Geometry: final body of the model. Coordinates: model frame, mm. A direction names the side the tool comes from. Coordinates: 2 decimals unless noted, no trailing zeros. Write each loop counter-clockwise with the first axis right and the second up, starting at its lowest first coordinate (ties: lowest second). Pieces come first, ordered by that corner, then holes. Notation, with made-up numbers: (-2, 62) -> (53, 62) arc R7 cw to (53, 73) -> close; hole circle Ø5 at (-9, 75.25). An arc over 180 degrees is marked (long way). One line per item, written item: value.
```python
from build123d import *
from build123d.topology import SkipClean

# Parameters (mm, degrees)
BOSS_EXTRUDE1_DEPTH     = 15
SKETCH2_R               = 30
BOSS_EXTRUDE2_DEPTH     = 25
SKETCH3_R               = 20
SKETCH3_R_2             = 10
BOSS_EXTRUDE3_DEPTH     = 15
CUT_EXTRUDE1_DEPTH      = 146.344418537
CUT_EXTRUDE1_DEPTH_BACK = 146.344418537
SKETCH4_R               = 20
SKETCH5_R               = 10
BOSS_EXTRUDE4_DEPTH     = 25


with BuildPart() as part:
    # Sketch1 → Boss-Extrude1 (new body)
    with BuildSketch(Plane.YZ):
        with BuildLine():
            Line((-14.764588704, 87.647058824), (-29.529177407, 5.294117647))
            ThreePointArc((-29.529177407, 5.294117647), (0, -30), (29.529177407, 5.294117647))
            Line((29.529177407, 5.294117647), (14.764588704, 87.647058824))
            ThreePointArc((14.764588704, 87.647058824), (0, 100), (-14.764588704, 87.647058824))
        make_face()
    extrude(amount=BOSS_EXTRUDE1_DEPTH)

    # Sketch2 → Boss-Extrude2 (add)
    with BuildSketch(Plane.YZ.offset(15)):
        with Locations(Location((0, 0, 0), (0, 0, 10.164248622))):
            Circle(SKETCH2_R)
    extrude(amount=BOSS_EXTRUDE2_DEPTH)

    # Sketch3 → Boss-Extrude3 (add)
    with SkipClean():  # the faces are left unmerged after this step: merging them gives an invalid solid
        with BuildSketch(Plane.YZ.offset(40)):
            with BuildLine():
                Line((6, 29.393876913), (78, 14.696938457))
                ThreePointArc((78, 14.696938457), (90, 0), (78, -14.696938457))
                Line((78, -14.696938457), (6, -29.393876913))
                ThreePointArc((6, -29.393876913), (-30, 0), (6, 29.393876913))
            make_face()
            with Locations(Location((0, 0, 0), (0, 0, 270))):
                Circle(SKETCH3_R, mode=Mode.SUBTRACT)
            with Locations(Location((75, 0, 0), (0, 0, 270))):
                Circle(SKETCH3_R_2, mode=Mode.SUBTRACT)
        extrude(amount=BOSS_EXTRUDE3_DEPTH)

    # Sketch4 → Cut-Extrude1 (cut, two sides: drawn at the far end of the back side and taken through both)
    with SkipClean():  # the faces are left unmerged after this step: merging them gives an invalid solid
        with BuildSketch(Plane.YZ.offset(55).offset(-CUT_EXTRUDE1_DEPTH_BACK)):
            with Locations(Location((0, 0, 0), (0, 0, 270))):
                Circle(SKETCH4_R)
        extrude(amount=CUT_EXTRUDE1_DEPTH + CUT_EXTRUDE1_DEPTH_BACK, mode=Mode.SUBTRACT)

    # Sketch5 → Boss-Extrude4 (add)
    with SkipClean():  # the faces are left unmerged after this step: merging them gives an invalid solid
        with BuildSketch(Plane(origin=(0, 0, 0), x_dir=(0, -1, 0), z_dir=(-1, 0, 0))):
            with Locations(Location((0, 85, 0), (0, 0, 270))):
                Circle(SKETCH5_R)
        extrude(amount=BOSS_EXTRUDE4_DEPTH)


solid = part.part
```
(1) Section A-A (y = 0). Return the cut outline in (x, z).
Responses:
outline: (-25, 75) -> (0, 75) -> (0, 20) -> (55, 20) -> (55, 30) -> (15, 30) -> (15, 100) -> (0, 100) -> (0, 95) -> (-25, 95) -> close; (0, -30) -> (55, -30) -> (55, -20) -> (0, -20) -> close
(2) Section B-B (z = 0). Return the cut outline in (x, y), then the cut area to 3 significant figures.
Responses:
outline: (0, -30) -> (55, -30) -> (55, -20) -> (0, -20) -> close; (0, 20) -> (55, 20) -> (55, 65) -> (40, 65) -> (40, 30) -> (0, 30) -> close; (40, 85) -> (55, 85) -> (55, 90) -> (40, 90) -> close
area: 1,700 mm2
(3) Line query: line 1 (Y direction, x = 43, z = 0); line 2 (Z direction, x = 22, y = 0); line 3 (X direction, y = 67.5, z = -7). Output: solid intervals per line, ascending. Write a range as [from, to].
Responses:
line 1: y = [-30, -20], [20, 65], [85, 90]
line 2: z = [-30, -20], [20, 30]
line 3: x = [40, 55]
(4) Section D-D (x = 42). Return the cut outline in (y, z), then the cut area to 3 significant figures.
Responses:
outline: (6, -29.39) -> (78, -14.7) arc R15 ccw to (78, 14.7) -> (6, 29.39) arc R30 ccw (long way) to start; hole circle Ø40 at (0, 0); hole circle Ø20 at (75, 0)
area: 3,640 mm2
(5) Pull-direction query (Y, two-part tool) for faces 4 (the cylindrical face through (47.395, 84.915, 1.302)), 5 (the cylindrical face through (-12, 0, 95)), 6 (the flat face through (15, 0, 53)); classes: released by +Y, released by -Y, zero draft, split by the parting line, or undercut.
Responses:
face 4: undercut
face 5: split by the parting line
face 6: zero draft
(6) Section C-C (x = 2.5). Return the cut outline in (y, z).
Responses:
outline: (-29.53, 5.29) arc R30 ccw (long way) to (29.53, 5.29) -> (14.76, 87.65) arc R15 ccw to (-14.76, 87.65) -> close; hole circle Ø40 at (0, 0)
(7) Reachability of faces 1 (the flat face through (47.395, 41.496, 22.148)), 2 (the cylindrical face through (27.115, -19.524, 4.336)), 3 (the flat face through (7.4, 22.25, 45.89)) from +Z, -Z, +X, -X, +Y, -Y: full face, straight path, thin tool, end or side. Return the list, or none.
Responses:
face 1: +Z, +X, +Y
face 2: +X, -X
face 3: +Z, -X, +Y
(8) First-contact query: pin 1 (8 mm diameter, centred on x = 22.5, z = 20.5, fed in from -Y); pin 2 (3 mm diameter, centred on x = 4, z = 73.5, fed in from +Y); pin 3 (4 mm diameter, centred on x = 23, y = 28.5, fed in from +Z). Flat tips, straight axial feed; report the tip coordinate or a pass-through.
Responses:
pin 1: stops at y = -25.05
pin 2: stops at y = 17.57
pin 3: stops at z = 14.06
